Here's the drawing with two shaded views (mm, measured from the low corner). I have some questions. A direction names the side the tool comes from. Coordinates: 2 decimals unless noted, no trailing zeros. Write each loop counter-clockwise with the first axis right and the second up, starting at its lowest first coordinate (ties: lowest second). Pieces come first, ordered by that corner, then holes.
Item 1: If we section it at B-B (x = 7.5): Please give me the cut outline in (y, z), then the cut area to 3 significant figures.
Item 2: If we section it at D-D (y = 7.5): Please give me the cut outline in (x, z), then the cut area to 3 significant figures.
Item 3: If I drill on line 1 (X direction, y = 8, z = 7.5); line 2 (Y direction, x = 9, z = 13.75), over which ranges is the centre line in solid material (lowest first)?
Item 4: If we section it at C-C (x = 10.25): Please give me the cut outline in (y, z).
Item 5: We'd pull the mould along Y, two halves only. Please class the marked faces 3, 4 and 5: +Y half, -Y half, draft (parallel to the pull), parting line (faces both ways), or undercut.
Item 6: For the marked faces 1 and 2, which set-ups out of +Z, -Z, +X, -X, +Y, -Y let a thin tool reach every point of the face, with its end or its side?
Item 7: If we section it at A-A (z = 7.5): Please give me the cut outline in (x, y), then the cut area to 3 significant figures.
Item 8: I'm going to push flat-ended pins straight in: pin 1 Ø1 at (y, z) = (6.5, 11) entering from -X; pin 2 Ø1.5 at (y, z) = (9, 10.5) entering from -X; pin 3 Ø5 at (x, y) = (12, 7.5) entering from -Z. Where does each tip first touch, or does it pass through?
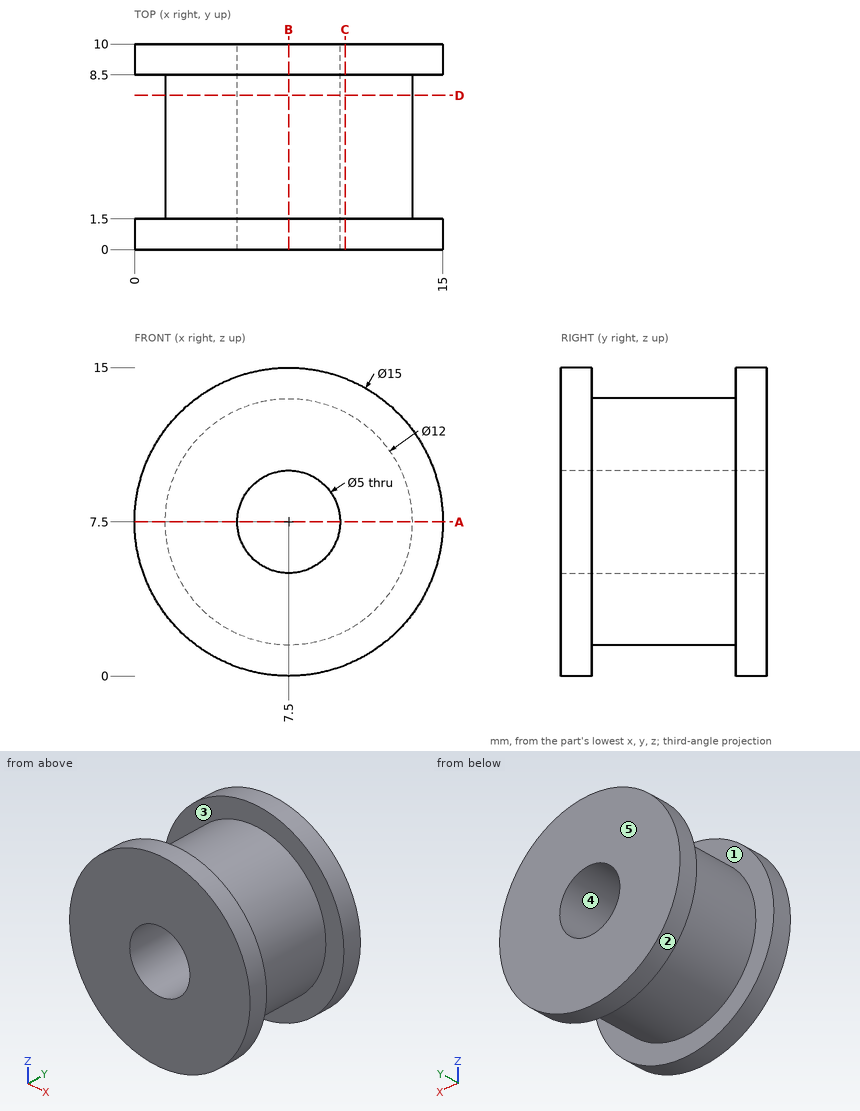
Answer list:
1. outline: (0, 0) - (1.5, 0) - (1.5, 1.5) - (8.5, 1.5) - (8.5, 0) - (10, 0) - (10, 5) - (0, 5) - close; (0, 10) - (10, 10) - (10, 15) - (8.5, 15) - (8.5, 13.5) - (1.5, 13.5) - (1.5, 15) - (0, 15) - close
1. area: 79.0 mm2
2. outline: circle Ø12 at (7.5, 7.5); hole circle Ø5 at (7.5, 7.5)
2. area: 93.5 mm2
3. line 1: x = 1.5 to 5, 10 to 13.5
3. line 2: y = 0 to 1.5, 8.5 to 10
4. outline: (0, 0.52) - (1.5, 0.52) - (1.5, 2.17) - (8.5, 2.17) - (8.5, 0.52) - (10, 0.52) - (10, 14.48) - (8.5, 14.48) - (8.5, 12.83) - (1.5, 12.83) - (1.5, 14.48) - (0, 14.48) - close
5. face 3: undercut
5. face 4: draft
5. face 5: +Y half
6. face 1: none
6. face 2: +Y, -Y
7. outline: (0, 0) - (5, 0) - (5, 10) - (0, 10) - (0, 8.5) - (1.5, 8.5) - (1.5, 1.5) - (0, 1.5) - close; (10, 0) - (15, 0) - (15, 1.5) - (13.5, 1.5) - (13.5, 8.5) - (15, 8.5) - (15, 10) - (10, 10) - close
7. area: 79.0 mm2
8. pin 1: stops at x = 2.3
8. pin 2: stops at x = 0.35
8. pin 3: stops at z = 0.33
